```python
from build123d import *

# Parameters (mm, degrees)
SKETCH1_R           = 12.1
BOSS_EXTRUDE1_DEPTH = 10.5
SKETCH2_R           = 2.5
CUT_EXTRUDE1_DEPTH  = 21.076603298
CHAMFER1_SIZE       = 2


with BuildPart() as part:
    # Sketch1 → Boss-Extrude1 (new body)
    with BuildSketch(Plane.XY):
        with Locations(Location((0, 0, 0), (0, 0, 180))):
            Circle(SKETCH1_R)
    extrude(amount=BOSS_EXTRUDE1_DEPTH)

    # Sketch2 → Cut-Extrude1 (cut, through all)
    with BuildSketch(Plane.XY.offset(10.5)):
        Circle(SKETCH2_R)
    extrude(amount=-CUT_EXTRUDE1_DEPTH, mode=Mode.SUBTRACT)

    # Chamfer1
    chamfer1_edges = [part.edges().sort_by_distance(p)[0] for p in [
        (12.1, 0, 0),
        (12.1, 0, 10.5),
    ]]
    chamfer(chamfer1_edges, length=CHAMFER1_SIZE)


solid = part.part
```
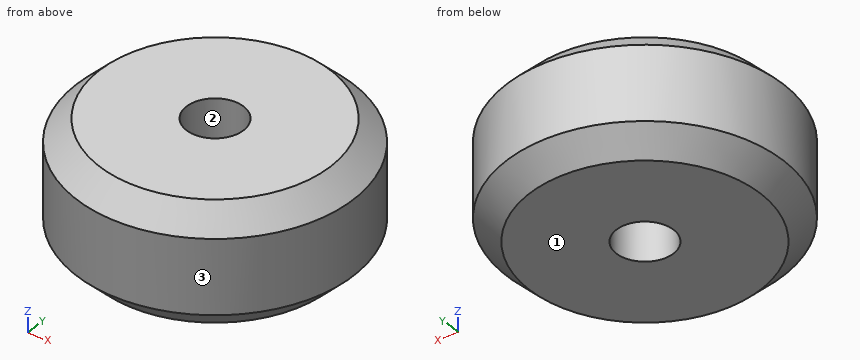
Design review of the part built by this model. Coordinates are the model's own, in mm. Face numbers are marked on the shaded views. Give positions to 0.01 mm unless a question says otherwise; leave off trailing zeros. Loops run counter-clockwise (first coordinate to the right, second up) from the corner with the lowest first, then second, coordinate; pieces in that order, holes last. Notation, with made-up numbers: M 62.5,5.25 L 102.5,5.25 A34 cw 102.5,42.25 Z; hole C 0.25,84 d7. An arc over 180 degrees is marked long. Return JSON: item names as keys, results as strings. Group by question number.
Item 1: For probe 1 along Y at (x, z) = (0, 7.75); probe 2 along Z at (x, y) = (-9.5, 5); probe 3 along X at (y, z) = (3.5, 6.5), list the stretches that pass through material, from the lowest coordinate up.
Item 2: We need section C-C (z = 8). Give the boundary of the cut face in (x, y), and give its area (3 significant figures).
Item 3: Insertion check: pin 1 Ø1.5 at (x, y) = (-6.5, 1.5) entering from -Z. The pin has a flat end and moves straight along its axis. Give the tip position at first contact, or say it passes through.
Item 4: We need section A-A (x = 0). Give the boundary of the cut face in (y, z).
Item 5: Mouldability with a two-part tool opening along Y and no side actions: class the marked faces 1, 2 and 3 as released by +Y, released by -Y, zero draft, split by the parting line, or undercut.
Output:
{
 "1": {"probe 1": "y = -12.1 to -2.5, 2.5 to 12.1", "probe 2": "z = 0.64 to 9.86", "probe 3": "x = -11.58 to 11.58"},
 "2": {"outline": "C 0,0 d24.2; hole C 0,0 d5", "area": "440 mm^2"},
 "3": {"pin 1": "stops at z = 0"},
 "4": {"outline": "M -12.1,2 L -10.1,0 L -2.5,0 L -2.5,10.5 L -10.1,10.5 L -12.1,8.5 Z; M 2.5,0 L 10.1,0 L 12.1,2 L 12.1,8.5 L 10.1,10.5 L 2.5,10.5 Z"},
 "5": {"face 1": "zero draft", "face 2": "undercut", "face 3": "split by the parting line"}
}
